```python
from build123d import *

# Parameters (mm, degrees)
BOSS_EXTRUDE1_DEPTH      = 150
BOSS_EXTRUDE1_DEPTH_BACK = 10
SKETCH1_R                = 15
SKETCH3_R                = 12.5
CUT_EXTRUDE2_DEPTH       = 105
CUT_EXTRUDE3_REACH       = 163.4
SKETCH4_R                = 10
CUT_EXTRUDE4_DEPTH       = 152.492574075
CUT_EXTRUDE4_DEPTH_BACK  = 152.492574075
SKETCH5_R                = 4
SKETCH6_W                = 5
SKETCH6_H                = 105
CUT_EXTRUDE12_DEPTH      = 152.492574194


with BuildPart() as part:
    # Sketch1 → Boss-Extrude1 (new, two sides: drawn at the far end of the back side and taken through both)
    with BuildSketch(Plane.XY.offset(-BOSS_EXTRUDE1_DEPTH_BACK)):
        Circle(SKETCH1_R)
    extrude(amount=BOSS_EXTRUDE1_DEPTH + BOSS_EXTRUDE1_DEPTH_BACK)

    # Sketch3 → Cut-Extrude2 (cut)
    with BuildSketch(Plane.XY.offset(125)):
        Circle(SKETCH3_R)
    extrude(amount=-CUT_EXTRUDE2_DEPTH, mode=Mode.SUBTRACT)

    # Sketch4 → Cut-Extrude3 (cut, up to next)
    with BuildSketch(Plane.XY.offset(150), mode=Mode.PRIVATE) as cut_extrude3_sk1:
        Circle(SKETCH4_R)
    cut_extrude3_tool1 = extrude(cut_extrude3_sk1.sketch, amount=-CUT_EXTRUDE3_REACH, mode=Mode.PRIVATE) & part.part
    add(cut_extrude3_tool1.solids().sort_by_distance((0, 0, 150))[0], mode=Mode.SUBTRACT)

    # Sketch5 → Cut-Extrude4 (cut, two sides: drawn at the far end of the back side and taken through both)
    with BuildSketch(Plane(origin=(0, 0, 0), x_dir=(1, 0, 0), z_dir=(0, 1, 0)).offset(-CUT_EXTRUDE4_DEPTH_BACK)):
        with Locations(Location((0, 0, 0), (0, 0, 270))):
            Circle(SKETCH5_R)
    extrude(amount=CUT_EXTRUDE4_DEPTH + CUT_EXTRUDE4_DEPTH_BACK, mode=Mode.SUBTRACT)

    # Sketch6 → Cut-Extrude12 (cut, through all)
    with BuildSketch(Plane(origin=(0, 0, 0), x_dir=(1, 0, 0), z_dir=(0, 1, 0))):
        with Locations((0, -72.5)):
            Rectangle(SKETCH6_W, SKETCH6_H)
    extrude(amount=CUT_EXTRUDE12_DEPTH, mode=Mode.SUBTRACT)


solid = part.part
```
Build history of the part. All positions in model axes, mm. A direction names the side the tool comes from. Round coordinates to 2 decimals unless told otherwise and drop trailing zeros. Write each loop counter-clockwise with the first axis right and the second up, starting at its lowest first coordinate (ties: lowest second). Pieces come first, ordered by that corner, then holes.
1) Pin check, flat tips, straight feed: pin 1 (15 mm diameter, centred on x = 0, y = 0, fed in from +Z); pin 2 (12 mm diameter, centred on y = 7, z = 58.5, fed in from -X); pin 3 (0.8 mm diameter, centred on y = 13, z = 79.5, fed in from -X). Stop position of each tip, or through.
2) Drill centre lines: probe 1 along Z at (x, y) = (6.5, -9); probe 2 along Z at (x, y) = (2, 11); probe 3 along Z at (x, y) = (-6, 1). Where is each one in solid material? Low to high.
3) Band-saw the part on B-B, the plane y = 5.5. List the corners of the cut face in (x, z), and give its area (3 significant figures).
4) Band-saw the part on C-C, the plane x = 6.5. List the corners of the cut face in (y, z), and give its area (3 significant figures).
5) Band-saw the part on A-A, the plane x = 0. List the corners of the cut face in (y, z), and give its area (3 significant figures).
6) Mould opens along X. For faces 1 (the cylindrical face through (-0.51, -12.49, 73.24)), 2 (the flat face through (0, 0, -10)), 3 (the cylindrical face through (6.92, -13.31, 68.88)) say: +X half, -X half, draft (parallel to the pull), parting line (faces both ways), or undercut.
7) 3-axis set-ups, long thin cutter, end or side, ignore diameter. For faces 4 (the flat face through (0, 1, 20)), 5 (the cylindrical face through (-3.905, -0.21, -0.867)), 6 (the flat face through (3, -10, 150)), 7 (the cylindrical face through (-2.17, -9.76, 137.68)), 8 (the flat face through (2.5, 14, 73)): which of +Z, -Z, +X, -X, +Y, -Y reach the whole face in a straight line?
8) Band-saw the part on D-D, the plane z = 76.5. List the corners of the cut face in (x, y), and give its area (3 significant figures).
Ans:
1. pin 1: stops at z = 20
1. pin 2: stops at x = -14.97
1. pin 3: stops at x = -8.14
2. probe 1: z = -10 to 20, 125 to 150
2. probe 2: z = -10 to -3.46, 3.46 to 20, 125 to 150
2. probe 3: z = -10 to 20
3. outline: (-13.96, -10) - (13.96, -10) - (13.96, 150) - (8.35, 150) - (8.35, 125) - (11.22, 125) - (11.22, 20) - (-11.22, 20) - (-11.22, 125) - (-8.35, 125) - (-8.35, 150) - (-13.96, 150) - close; hole circle Ø8 at (0, 0)
3. area: 1,640 mm2
4. outline: (-13.52, -10) - (13.52, -10) - (13.52, 150) - (7.6, 150) - (7.6, 125) - (10.68, 125) - (10.68, 20) - (-10.68, 20) - (-10.68, 125) - (-7.6, 125) - (-7.6, 150) - (-13.52, 150) - close
4. area: 1,700 mm2
5. outline: (-15, -10) - (15, -10) - (15, -4) - (-15, -4) - close; (-15, 4) - (15, 4) - (15, 20) - (-12.5, 20) - (-12.5, 125) - (-10, 125) - (-10, 150) - (-15, 150) - close; (10, 125) - (15, 125) - (15, 150) - (10, 150) - close
5. area: 1,170 mm2
6. face 1: undercut
6. face 2: draft
6. face 3: parting line
7. face 4: none
7. face 5: +Y, -Y
7. face 6: +Z, +X, -X, +Y, -Y
7. face 7: +Z
7. face 8: +Y
8. outline: (-2.5, 12.25) - (-2.5, 14.79) arc R15 ccw (long way) to (2.5, 14.79) - (2.5, 12.25) arc R12.5 cw (long way) to start
8. area: 203 mm2
